Source: CAD feature listing. Evaluate the final solid. Frame: model axes, mm. A direction names the side the tool comes from. Round coordinates to 2 decimals unless told otherwise and drop trailing zeros. Write each loop counter-clockwise with the first axis right and the second up, starting at its lowest first coordinate (ties: lowest second). Pieces come first, ordered by that corner, then holes.
```python
from build123d import *

# Parameters (mm, degrees)
BOSS_EXTRUDE1_DEPTH = 6.35


with BuildPart() as part:
    # Sketch1 → Boss-Extrude1 (new body)
    with BuildSketch(Plane(origin=(0, 0, 0), x_dir=(1, 0, 0), z_dir=(0, 1, 0))):
        Polygon((-38.1, -38.1), (38.1, -38.1), (38.1, 38.1), (-38.1, 38.1), (-38.1, 24.13), (-46.2026, 24.13), (-46.2026, 20.447), (-44.0944, 20.447), (-44.0944, 17.78), (-51.9684, 17.78), (-51.9684, 20.447), (-49.8602, 20.447), (-49.8602, 24.13), (-57.9628, 24.13), (-57.9628, 9.9314), (-38.1, 9.9314), (-38.1, -9.9314), (-57.9628, -9.9314), (-57.9628, -24.13), (-49.8602, -24.13), (-49.8602, -20.447), (-51.9684, -20.447), (-51.9684, -17.78), (-44.0944, -17.78), (-44.0944, -20.447), (-46.2026, -20.447), (-46.2026, -24.13), (-38.1, -24.13), align=None)
        with BuildLine():
            Line((7.227071664, -18.99759929), (12.838867764, -15.757627301))
            Line((12.838867764, -15.757627301), (11.99371709, -14.293783392))
            ThreePointArc((11.99371709, -14.293783392), (16.159242555, 9.329543039), (-6.381920989, 17.533755382))
            Line((-6.381920989, 17.533755382), (-7.227071664, 18.99759929))
            Line((-7.227071664, 18.99759929), (-12.838867764, 15.757627301))
            Line((-12.838867764, 15.757627301), (-11.99371709, 14.293783392))
            ThreePointArc((-11.99371709, 14.293783392), (-16.159242555, -9.329543039), (6.381920989, -17.533755382))
            Line((6.381920989, -17.533755382), (7.227071664, -18.99759929))
        make_face(mode=Mode.SUBTRACT)
    extrude(amount=-BOSS_EXTRUDE1_DEPTH)


solid = part.part
```
Q1. Section query A-A, the plane x = 3. Output: boundary loops of the cut face in (y, z), and give its area (3 significant figures).
Q2. Mould query, pull axis X, two halves, no side actions, for faces 4 (the face through (-46.203, -3, -22)), 5 (the face through (-48, -3, 9.931)), 6 (the face through (-57.963, -3, 17)), 7 (the face through (-16.34, -3.13, 9.01)). Classes: pulls with the +X half, pulls with the -X half, needs draft (parallel to the pull), parting line crosses it, or undercut.
Q3. Line query: line 1 (Z direction, x = -45.5, y = -4.5); line 2 (X direction, y = -5.25, z = -21.5); line 3 (X direction, y = -4.5, z = 6). Output: solid intervals per line, ascending.
Q4. Set-up query: faces 1 (the face through (-38.1, -3, 31)), 2 (the face through (-45, -3, -20.447)), 3 (the face through (-48, -3, -9.931)). Return all of +Z, -Z, +X, -X, +Y, -Y with unobstructed straight access to the full face (end or side cutting, diameter ignored); none if empty.
Q5. Pin query (flat end, axial travel): P1, Ø3, axis at x = -49, y = -3, coming from the +Z side; P2, Ø1.1, axis at x = -50.5, y = -3, coming from the -Z side; P3, Ø1.9, axis at y = -2.5, z = -31, coming from the -X side. Return the tip coordinate at first contact, or that it passes through.
Q6. Section query B-B, the plane z = -30.5. Output: boundary loops of the cut face in (x, y), and give its area (3 significant figures).
Filled in:
1. outline: (-6.35, -38.1) - (0, -38.1) - (0, -18.42) - (-6.35, -18.42) - close; (-6.35, 18.42) - (0, 18.42) - (0, 38.1) - (-6.35, 38.1) - close
1. area: 250 mm2
2. face 4: undercut
2. face 5: needs draft
2. face 6: pulls with the -X half
2. face 7: undercut
3. line 1: z = -24.13 to -20.45, -17.78 to -9.93, 9.93 to 17.78, 20.45 to 24.13
3. line 2: x = -57.96 to -49.86, -46.2 to 38.1
3. line 3: x = -38.1 to -17.67, 17.67 to 38.1
4. face 1: +Z, -X, +Y, -Y
4. face 2: +Y, -Y
4. face 3: -X, +Y, -Y
5. P1: stops at z = 24.13
5. P2: stops at z = -24.13
5. P3: stops at x = -38.1
6. outline: (-38.1, -6.35) - (38.1, -6.35) - (38.1, 0) - (-38.1, 0) - close
6. area: 484 mm2
